Part model, mm, in its own coordinate system. Coordinates: 2 decimals unless noted, no trailing zeros. Loops run counter-clockwise (first coordinate to the right, second up) from the corner with the lowest first, then second, coordinate; pieces in that order, holes last. Notation, with made-up numbers: (74.5, 42.25) - (97.5, 42.25) arc R23 ccw to (97.5, 52.25) - close; hole circle Ø4 at (-7.5, 29.25). An arc over 180 degrees is marked (long way). Use a Markdown table: item, result. Add a question column.
1. Pull direction X, two halves, no side cores. Call faces 1 (the cylindrical face through (-11.9, 1.59, -1.43)), 2 (the cylindrical face through (-8.19, 1.59, 64.28)), 3 (the cylindrical face through (-4.57, 1.59, 67.4)): pulls with the +X half, pulls with the -X half, needs draft (parallel to the pull), parting line crosses it, or undercut.
2. Band-saw the part on B-B, the plane y = 1.35. Give the cut face in (x, z).
3. Band-saw the part on C-C, the plane x = -8.25. Give the cut face in (y, z).
4. Band-saw the part on A-A, the plane z = 1. Give the cut face in (x, y), plus the area to 3 significant figures.
5. Wall check: probe 1 along X at (y, z) = (0.7, 1); probe 2 along Z at (x, y) = (-7.25, 1.1); probe 3 along Z at (x, y) = (-9.5, 0.4). Give the ranges that are in metal, low to high. Write a range as [from, to].
from build123d import *

# Parameters (mm, degrees)
BOSS_EXTRUDE1_DEPTH = 3.14
SKETCH7_R           = 1.47
CUT_EXTRUDE1_DEPTH  = 70.210617683
SKETCH8_W           = 16.5
SKETCH8_H           = 4
CUT_EXTRUDE2_DEPTH  = 70.210617683
FILLET1_R           = 2
SKETCH9_R           = 1.47
CUT_EXTRUDE3_DEPTH  = 70.210617683


with BuildPart() as part:
    # Sketch1 → Boss-Extrude1 (new body)
    with BuildSketch(Plane(origin=(0, 0, 0), x_dir=(1, 0, 0), z_dir=(0, 1, 0))):
        Polygon((12.5, 2), (12.5, -2), (-4, -2), (-4, -68), (-12.5, -68), (-12.5, 2), (-8.5, 2), align=None)
    extrude(amount=BOSS_EXTRUDE1_DEPTH)

    # Sketch7 → Cut-Extrude1 (cut, through all)
    with BuildSketch(Plane(origin=(0, 3.14, 0), x_dir=(1, 0, 0), z_dir=(0, 1, 0))):
        with Locations(Location((-8.25, -65.75, 0), (0, 0, 270))):
            Circle(SKETCH7_R)
    extrude(amount=-CUT_EXTRUDE1_DEPTH, mode=Mode.SUBTRACT)

    # Sketch8 → Cut-Extrude2 (cut, through all)
    with BuildSketch(Plane.XZ):
        with Locations((4.25, 0)):
            Rectangle(SKETCH8_W, SKETCH8_H)
    extrude(amount=-CUT_EXTRUDE2_DEPTH, mode=Mode.SUBTRACT)

    # Fillet1
    fillet1_edges = [part.edges().sort_by_distance(p)[0] for p in [
        (-4, 1.57, 68),
        (-12.5, 1.57, 68),
        (-12.5, 1.57, -2),
        (-4, 1.57, -2),
    ]]
    fillet(fillet1_edges, radius=FILLET1_R)

    # Sketch9 → Cut-Extrude3 (cut, through all)
    with BuildSketch(Plane.XZ):
        with Locations(Location((-8.25, 1, 0), (0, 0, 270))):
            Circle(SKETCH9_R)
    extrude(amount=-CUT_EXTRUDE3_DEPTH, mode=Mode.SUBTRACT)


solid = part.part
Geometry check:
| question | item | result |
|---|---|---|
| 1 | face 1 | pulls with the -X half |
| 1 | face 2 | undercut |
| 1 | face 3 | pulls with the +X half |
| 2 | outline | (-12.5, 0) arc R2 ccw to (-10.5, -2) - (-6, -2) arc R2 ccw to (-4, 0) - (-4, 66) arc R2 ccw to (-6, 68) - (-10.5, 68) arc R2 ccw to (-12.5, 66) - close; hole circle Ø2.94 at (-8.25, 1); hole circle Ø2.94 at (-8.25, 65.75) |
| 3 | outline | (0, -2) - (3.14, -2) - (3.14, -0.47) - (0, -0.47) - close; (0, 2.47) - (3.14, 2.47) - (3.14, 64.28) - (0, 64.28) - close; (0, 67.22) - (3.14, 67.22) - (3.14, 68) - (0, 68) - close |
| 4 | outline | (-12.5, 0) - (-9.72, 0) - (-9.72, 3.14) - (-12.5, 3.14) - close; (-6.78, 0) - (-4, 0) - (-4, 3.14) - (-6.78, 3.14) - close |
| 4 | area | 17.5 mm^2 |
| 5 | probe 1 | x = [-12.5, -9.72], [-6.78, -4] |
| 5 | probe 2 | z = [-2, -0.08], [2.08, 64.67], [66.83, 68] |
| 5 | probe 3 | z = [-2, 0.23], [1.77, 64.98], [66.52, 68] |
